Autodesk Inventor part; units mm, degrees
ref_plane "YZ Plane" through (0, 0, 0) normal (1, 0, 0) x (0, 1, 0)
ref_plane "XZ Plane" through (0, 0, 0) normal (0, 1, 0) x (-1, 0, 0)
ref_plane "XY Plane" through (0, 0, 0) normal (0, 0, 1) x (1, 0, 0)
sketch "Sketch1" plane through (0, 0, 0) normal (0, 0, 1) x (1, 0, 0)
  line L0 (-60, -60) -> (60, -60)
  line L1 (60, -60) -> (60, 60)
  line L2 (60, 60) -> (-60, 60)
  line L3 (-60, 60) -> (-60, -60)
  line L4 (-60, -60) -> (60, 60) construction
  line L5 (60, -60) -> (-60, 60) construction
  point P0 (0, 0)
  dimension "d0" = 120
  dimension "d1" = 120
extrude "Extrusion1" add sketch "Sketch1" along normal blind 3.175
sketch "Sketch5" plane through (0, 0, 3.175) normal (0, 0, 1) x (1, 0, 0)
  line L0 (-60, -60) -> (60, -60)
  line L1 (60, -60) -> (60, 60)
  line L2 (60, 60) -> (-60, 60)
  line L3 (-60, 60) -> (-60, -60)
  line L4 (-60, -60) -> (60, -60)
  line L5 (55, -60) -> (45, -60)
  line L6 (45, -60) -> (45, -56.825)
  line L7 (45, -56.825) -> (55, -56.825)
  line L8 (55, -56.825) -> (55, -60)
  point P0 (0, 0)
  dimension "d25" = 10
  dimension "d27" = 5
  dimension "d41" = 3.175
extrude "Extrusion3" cut sketch "Sketch5" against normal up to surface (3.175 mm away) contours L6 L7 L8 L0
pattern_linear "Rectangular Pattern2" count 6 spacing 20 along (-1, 0, 0) of "Extrusion3"
mirror "Mirror2" about plane through (0, 0, 0) normal (0, 1, 0) of "Extrusion3", "Rectangular Pattern2"
sketch "Sketch6" plane through (0, 0, 3.175) normal (0, 0, 1) x (1, 0, 0)
  line L0 (-60, -60) -> (-55, -60)
  line L1 (-45, -60) -> (-35, -60)
  line L2 (-25, -60) -> (-15, -60)
  line L3 (-5, -60) -> (5, -60)
  line L4 (15, -60) -> (25, -60)
  line L5 (35, -60) -> (45, -60)
  line L6 (60, -60) -> (60, 60)
  line L7 (60, 60) -> (55, 60)
  line L8 (45, 60) -> (35, 60)
  line L9 (25, 60) -> (15, 60)
  line L10 (5, 60) -> (-5, 60)
  line L11 (-15, 60) -> (-25, 60)
  line L12 (-35, 60) -> (-45, 60)
  line L13 (-60, 60) -> (-60, -60)
  line L14 (-60, -55) -> (-56.825, -55)
  line L15 (-56.825, -55) -> (-56.825, -45)
  line L16 (-56.825, -45) -> (-60, -45)
  line L17 (-60, -45) -> (-60, -55)
  line L18 (55, -60) -> (60, -60)
  line L19 (-55, 60) -> (-60, 60)
  line L20 (-55, 56.825) -> (-55, 60)
  line L21 (-55, -60) -> (-55, -56.825)
  line L22 (-55, -56.825) -> (-45, -56.825)
  line L23 (-45, -56.825) -> (-45, -60)
  line L24 (-35, -60) -> (-35, -56.825)
  line L25 (-35, -56.825) -> (-25, -56.825)
  line L26 (-25, -56.825) -> (-25, -60)
  line L27 (-15, -60) -> (-15, -56.825)
  line L28 (-15, -56.825) -> (-5, -56.825)
  line L29 (-5, -56.825) -> (-5, -60)
  line L30 (5, -60) -> (5, -56.825)
  line L31 (5, -56.825) -> (15, -56.825)
  line L32 (15, -56.825) -> (15, -60)
  line L33 (25, -60) -> (25, -56.825)
  line L34 (25, -56.825) -> (35, -56.825)
  line L35 (35, -56.825) -> (35, -60)
  line L36 (45, -60) -> (45, -56.825)
  line L37 (45, -56.825) -> (55, -56.825)
  line L38 (55, -56.825) -> (55, -60)
  line L39 (55, 60) -> (55, 56.825)
  line L40 (55, 56.825) -> (45, 56.825)
  line L41 (45, 56.825) -> (45, 60)
  line L42 (35, 60) -> (35, 56.825)
  line L43 (35, 56.825) -> (25, 56.825)
  line L44 (25, 56.825) -> (25, 60)
  line L45 (15, 60) -> (15, 56.825)
  line L46 (15, 56.825) -> (5, 56.825)
  line L47 (5, 56.825) -> (5, 60)
  line L48 (-5, 60) -> (-5, 56.825)
  line L49 (-5, 56.825) -> (-15, 56.825)
  line L50 (-15, 56.825) -> (-15, 60)
  line L51 (-25, 60) -> (-25, 56.825)
  line L52 (-25, 56.825) -> (-35, 56.825)
  line L53 (-35, 56.825) -> (-35, 60)
  line L54 (-45, 60) -> (-45, 56.825)
  line L55 (-45, 56.825) -> (-55, 56.825)
  point P0 (0, 0)
  dimension "d34" = 10
  dimension "d35" = 5
  dimension "d42" = 3.175
extrude "Extrusion4" cut sketch "Sketch6" against normal up to surface (3.175 mm away) contours L13 L16 L15 L14
pattern_linear "Rectangular Pattern3" count 6 spacing 20 along (0, 1, 0) of "Extrusion4"
mirror "Mirror3" about plane through (0, 0, 0) normal (1, 0, 0) of "Extrusion4", "Rectangular Pattern3"
equation "\"d0\" = width"
equation "\"d1\" = depth"
equation "\"d2\" = materialThickness"
equation "\"d25\" = notchWidth"
equation "\"d27\" = 0 * materialThickness + 0.5 * width - 5.5 * notchWidth"
equation "\"d41\" = materialThickness"
equation "\"d32\" = 2 * notchWidth"
equation "\"d34\" = notchWidth"
equation "\"d35\" = 0 * materialThickness + 0.5 * depth - 5.5 * notchWidth"
equation "\"d42\" = materialThickness"
equation "\"d40\" = 2 * notchWidth"
equation "\"width\" = 120"
equation "\"depth\" = 120"
equation "\"materialThickness\" = 3.175"
equation "\"laserKerf\" = 0.12"
equation "\"cardPinDiameter\" = 3"
equation "\"cardFillet\" = 2.88"
equation "\"cardSelected\" = 1"
equation "\"cardThickness\" = 0.76"
equation "\"cardHeight\" = 53.98"
equation "\"cardWidth\" = 85.6"
equation "\"centeralShaftDiameter\" = 8"
equation "\"cardClearence\" = 0.5"
equation "\"bearingOd\" = 22"
equation "\"bearingWidth\" = 8"
equation "\"axleHeight\" = 95"
equation "\"nutTrapDepth\" = 2.5"
equation "\"nutTrapwidth\" = 5.5"
equation "\"nutTrapClearence\" = 2"
equation "\"magnetLength\" = 3"
equation "\"magnetDiameter\" = 6"
equation "\"magnetProtusion\" = 0.25"
equation "\"notchWidth\" = 10"
equation "\"spoolThickness\" = 5.588"
properties part number "topBottomPanel" material "Polycarbonate, Clear"
Can you work these out from the model? Positions are in its coordinate system, mm. A direction names the side the tool comes from. Round coordinates to 2 decimals unless told otherwise and drop trailing zeros. Loops run counter-clockwise (first coordinate to the right, second up) from the corner with the lowest first, then second, coordinate; pieces in that order, holes last. Notation, with made-up numbers: (-8.75, -8.5) -> (32.25, -8.5) arc R18 ccw to (32.25, 23.5) -> close; hole circle Ø9 at (88.5, 85.25). An arc over 180 degrees is marked (long way). One line per item, written item: value. Start each with the question number.
1. For pin 1 (1.5 mm diameter, centred on x = 17, y = -4, fed in from -Z); pin 2 (1 mm diameter, centred on y = 49, z = 1, fed in from -X) (3 decimals); pin 3 (1 mm diameter, centred on y = 30, z = 2, fed in from +X) (3 decimals), each with a flat end and sliding along its axis, tell me the tip position at first contact or that it passes through.
2. If we section it at A-A, the plane y = 52: Write out the boundary of the cut face in (x, z) (3 decimals), then the cut area to 3 significant figures.
3. If I drill on probe 1 along X at (y, z) = (-6.5, 0.25) (3 decimals), over which ranges is the centre line in solid material (lowest first)?
4. For faces 4 (the flat face through (45, -58, 2)), 5 (the flat face through (58, -45, 2)), 6 (the flat face through (-58, -15, 2)), 7 (the flat face through (-35, 58, 2)), which set-ups out of +Z, -Z, +X, -X, +Y, -Y let a thin tool reach every point of the face, with its end or its side?
5. If we mould it in two halves opening along Y, with no side actions, what happens to faces 1 (the flat face through (55, -58, 2)), 2 (the flat face through (58, 35, 2)), 3 (the flat face through (30, -56.825, 2))? For each: pulls with the +Y half, pulls with the -Y half, needs draft (parallel to the pull), parting line crosses it, or undercut.
Calculated:
1. pin 1: stops at z = 0
1. pin 2: stops at x = -56.825
1. pin 3: stops at x = 56.825
2. outline: (-56.825, 0) -> (56.825, 0) -> (56.825, 3.175) -> (-56.825, 3.175) -> close
2. area: 361 mm²
3. probe 1: x = -56.825 to 56.825
4. face 4: +Z, -Z, -Y
4. face 5: +Z, -Z, +X
4. face 6: +Z, -Z, -X
4. face 7: +Z, -Z, +Y
5. face 1: needs draft
5. face 2: undercut
5. face 3: pulls with the -Y half
